Autodesk Inventor part; units mm, degrees
ref_plane "YZ Plane" through (0, 0, 0) normal (1, 0, 0) x (0, 1, 0)
ref_plane "XZ Plane" through (0, 0, 0) normal (0, 1, 0) x (-1, 0, 0)
ref_plane "XY Plane" through (0, 0, 0) normal (0, 0, 1) x (1, 0, 0)
sketch "Sketch1" plane through (0, 0, 0) normal (0, 1, 0) x (-1, 0, 0)
  line L0 (102.5, 187.5) -> (-102.5, 187.5)
  line L1 (-102.5, 187.5) -> (-102.5, -187.5)
  line L2 (-102.5, -187.5) -> (102.5, -187.5)
  line L3 (102.5, -187.5) -> (102.5, 187.5)
  line L4 (102.5, 187.5) -> (-102.5, -187.5) construction
  line L5 (-102.5, 187.5) -> (102.5, -187.5) construction
  point P0 (0, 0)
  dimension "d0" = 205
  dimension "d1" = 375
extrude "Extrusion1" add sketch "Sketch1" along normal blind 10
fillet "Fillet1" radius 1 2 edges at (102.5, 10, 0) (-102.5, 10, 0)
sketch "Sketch3" plane through (0, 0, 0) normal (0, -1, 0) x (1, 0, 0)
  line L0 (102.5, -187.5) -> (-102.5, -187.5)
  line L1 (102.5, 187.5) -> (102.5, -187.5)
  line L2 (-102.5, 187.5) -> (102.5, 187.5)
  line L3 (-102.5, -187.5) -> (-102.5, 187.5)
  line L4 (102.5, 187.5) -> (102.5, -187.5)
  line L5 (-102.5, -187.5) -> (-102.5, 187.5)
  line L6 (102.5, 187.5) -> (-102.5, 187.5)
  line L7 (-102.5, 187.5) -> (-102.5, 177.5)
  line L8 (-102.5, 177.5) -> (102.5, 177.5)
  line L9 (102.5, 177.5) -> (102.5, 187.5)
  line L10 (102.5, 182.5) -> (77.5, 182.5)
  line L11 (77.5, 182.5) -> (0, 182.5)
  line L12 (0, 182.5) -> (-77.5, 182.5)
  circle A0 centre (77.5, 182.5) radius 3.3
  circle A1 centre (0, 182.5) radius 3.3
  circle A2 centre (-77.5, 182.5) radius 3.3
  point P0 (0, 0)
  dimension "d5" = 10
  dimension "d21" = 25
  dimension "d22" = 77.5
  dimension "d23" = 6.6
  dimension "d24" = 6.6
  dimension "d25" = 6.6
extrude "Extrusion2" cut sketch "Sketch3" against normal up to surface (10 mm away) contours A2 | A1 L12 L11 | L11 L12 A1 | A0 L11 L10 | L10 L11 A0
sketch "Sketch4" plane through (0, 10, 0) normal (0, 1, 0) x (1, 0, 0)
  line L0 (-101.5, -187.5) -> (-102.5, -187.5)
  line L1 (-102.5, -187.5) -> (-18.3, -187.5)
  line L2 (-101.5, -187.5) -> (101.5, -187.5)
  line L3 (-18.3, -187.5) -> (-18.3, -27.5)
  circle A0 centre (-18.3, -27.5) radius 7.5
  line L4 (-18.3, -27.5) -> (-18.3, 92.5)
  circle A1 centre (-18.3, 92.5) radius 10
  circle A2 centre (77.5, -182.5) radius 3.3
  circle A3 centre (-77.5, -182.5) radius 3.3
  circle A4 centre (0, -182.5) radius 3.3
  line L5 (-101.5, -187.5) -> (-101.5, 187.5)
  line L6 (-101.5, -187.5) -> (101.5, -187.5)
  line L7 (101.5, 187.5) -> (101.5, -187.5)
  line L8 (101.5, 187.5) -> (-101.5, 187.5)
  line L9 (101.5, 187.5) -> (-101.5, 187.5)
  line L10 (0, 187.5) -> (0, -187.5)
  circle A5 centre (18.3, -27.5) radius 7.5
  circle A6 centre (18.3, 92.5) radius 10
  point P0 (0, 0)
  dimension "d11" = 84.2
  dimension "d12" = 160
  dimension "d13" = 15
  dimension "d16" = 120
  dimension "d17" = 20
extrude "Extrusion3" cut sketch "Sketch4" against normal up to surface (10 mm away) contours A5 | A6
properties part number "płyta_boczna_obudowy_odbita"
Check sheet for the modelled part. Datum: model origin and axes. Units: mm. Give positions to 0.01 mm unless a question says otherwise; leave off trailing zeros. Order: outer loops, then holes, each group sorted by start corner. A loop starts at its lowest first (then second) coordinate and runs counter-clockwise, first axis right, second up. Notation, with made-up numbers: M -5,-32.75 L 31,-32.75 A7 cw 31,-20.75 Z; hole C 46.5,48.5 d7. An arc over 180 degrees is marked long. Answer in a Markdown table with one row per item. Add a question column.
Q1. Thickness scan on L1, parallel to Z at x = 18.3, y = 8; L2, parallel to X at y = 7, z = 182.5; L3, parallel to Z at x = 0, y = 2.75. Record the ranges inside material, lowest first.
Q2. Sectioned sample at A-A, the plane z = 27.5. Record the boundary of the cut face in (x, y), and give its area (3 significant figures).
Q3. Sectioned sample at B-B, the plane x = 18.3. Record the boundary of the cut face in (y, z), and give its area (3 significant figures).
Q4. Sectioned sample at C-C, the plane z = -92.5. Record the boundary of the cut face in (x, y), and give its area (3 significant figures).
Q5. Release check for a two-part mould opening along Z. For faces 1 (the cylindrical face through (-0.72, 4.93, 179.28)), 2 (the flat face through (1, 5, -187.5)), 3 (the flat face through (1, 10, 3)) record: released by +Z, released by -Z, zero draft, split by the parting line, or undercut.
Verdict:
| question | item | result |
|---|---|---|
| 1 | L1 | -187.5 to -102.5, -82.5 to 20, 35 to 187.5 |
| 1 | L2 | -102.5 to -80.8, -74.2 to -3.3, 3.3 to 74.2, 80.8 to 102.5 |
| 1 | L3 | -187.5 to 179.2, 185.8 to 187.5 |
| 2 | outline | M -102.5,0 L 10.8,0 L 10.8,10 L -101.5,10 A1 ccw -102.5,9 Z; M 25.8,0 L 102.5,0 L 102.5,9 A1 ccw 101.5,10 L 25.8,10 Z |
| 2 | area | 1,900 mm² |
| 3 | outline | M 0,-187.5 L 10,-187.5 L 10,-102.5 L 0,-102.5 Z; M 0,-82.5 L 10,-82.5 L 10,20 L 0,20 Z; M 0,35 L 10,35 L 10,187.5 L 0,187.5 Z |
| 3 | area | 3,400 mm² |
| 4 | outline | M -102.5,0 L 8.3,0 L 8.3,10 L -101.5,10 A1 ccw -102.5,9 Z; M 28.3,0 L 102.5,0 L 102.5,9 A1 ccw 101.5,10 L 28.3,10 Z |
| 4 | area | 1,850 mm² |
| 5 | face 1 | undercut |
| 5 | face 2 | released by -Z |
| 5 | face 3 | zero draft |
